Source: CAD feature listing. Evaluate the final solid. Frame: model axes, mm. A direction names the side the tool comes from. Give positions to 0.01 mm unless a question says otherwise; leave off trailing zeros. Write each loop counter-clockwise with the first axis right and the second up, starting at its lowest first coordinate (ties: lowest second). Pieces come first, ordered by that corner, then holes. Notation, with made-up numbers: (-23, -11) - (-11, -11) arc R9 ccw to (-11, -7) - close; hole circle Ø2 at (64, -3.75). An arc over 180 degrees is marked (long way). One line per question, with ' | ' between items. Start each with the question number.
(1) Ray query, line 1 (Y direction, x = 15, z = 4); line 2 (X direction, y = 5, z = 6.25); line 3 (X direction, y = 12, z = 4). Return the intervals inside material, ascending. Write a range as [from, to].
(2) Section B-B, the plane x = 55. Return loops of the section in (y, z), plus the area to 3 significant figures.
(3) Section D-D, the plane y = 12.5. Return loops of the section in (x, z), plus the area to 3 significant figures.
(4) Section C-C, the plane y = 49. Return loops of the section in (x, z).
(5) Pin query (flat end, axial travel): pin 1 (19 mm diameter, centred on x = 33.93, y = 49, fed in from -Z); pin 2 (16 mm diameter, centred on x = 55, y = 15, fed in from -Z). Return the tip coordinate at first contact, or that it passes through.
(6) Access query for faces 4 (the flat face through (31, 8, 2)), 5 (the flat face through (17, 10, 8)), 6 (the cylindrical face through (55, 31, 2)). Directions: +Z, -Z, +X, -X, +Y, -Y. A direction counts if a zero-diameter tool reaches every point of the face in a straight line with its end or side. Return the directions, or none.
(7) Section A-A, the plane z = 1.5. Return loops of the section in (x, y).
(8) Draft query along X for faces 1 (the flat face through (-1, 27, 7)), 2 (the flat face through (34, 70, 8)), 3 (the flat face through (39, 7, 2)). Return one class per face: +X half, -X half, draft (parallel to the pull), parting line (faces both ways), or undercut.
```python
from build123d import *

# Parameters (mm, degrees)
SKETCH1_W               = 70
SKETCH1_H               = 70
BOSS_EXTRUDE1_DEPTH     = 10
SKETCH2_R               = 12
SKETCH2_R_2             = 2
SKETCH2_R_3             = 11.5
CUT_EXTRUDE1_DEPTH      = 10
SKETCH3_W               = 10
SKETCH3_H               = 70
BOSS_EXTRUDE2_DEPTH     = 15
SKETCH4_W               = 10
SKETCH4_H               = 70
BOSS_EXTRUDE3_DEPTH     = 15
SKETCH5_R               = 11.5
SKETCH5_R_2             = 4
BOSS_EXTRUDE4_DEPTH     = 2
SKETCH6_R               = 1.5
SKETCH6_R_2             = 1.648708122
CUT_EXTRUDE3_DEPTH      = 10
BOSS_EXTRUDE5_START     = -10
SKETCH7_R               = 11.986708095
SKETCH7_R_2             = 2
BOSS_EXTRUDE5_DEPTH     = 10
SKETCH8_R               = 12
CUT_EXTRUDE4_DEPTH      = 10
SKETCH9_R               = 2
CUT_EXTRUDE5_DEPTH      = 10
CUT_EXTRUDE7_DEPTH      = 5
SKETCH15_W              = 14
SKETCH15_H              = 70
CUT_EXTRUDE8_DEPTH      = 5
CUT_EXTRUDE9_DEPTH      = 19
CUT_EXTRUDE9_DEPTH_BACK = 48
SKETCH16_R              = 1.5
SKETCH17_R              = 5
CUT_EXTRUDE10_DEPTH     = 19
SKETCH18_R              = 16.289174866
SKETCH18_R_2            = 12
BOSS_EXTRUDE6_DEPTH     = 5


with BuildPart() as part:
    # Sketch1 → Boss-Extrude1 (new body)
    with BuildSketch(Plane.XY):
        with Locations((35, 35)):
            Rectangle(SKETCH1_W, SKETCH1_H)
    extrude(amount=BOSS_EXTRUDE1_DEPTH)

    # Sketch2 → Cut-Extrude1 (cut)
    with BuildSketch(Plane.XY.offset(10)):
        with Locations((35, 49)):
            Circle(SKETCH2_R)
        with Locations((19.5, 65)):
            Circle(SKETCH2_R_2)
        with Locations((50.5, 65)):
            Circle(SKETCH2_R_2)
        with Locations((19.5, 34)):
            Circle(SKETCH2_R_2)
        with Locations((50.5, 34)):
            Circle(SKETCH2_R_2)
        with Locations((15, 15)):
            Circle(SKETCH2_R_3)
        with Locations((55, 15)):
            Circle(SKETCH2_R_3)
    extrude(amount=-CUT_EXTRUDE1_DEPTH, mode=Mode.SUBTRACT)

    # Sketch3 → Boss-Extrude2 (add)
    with BuildSketch(Plane.ZY):
        with Locations((5, 35)):
            Rectangle(SKETCH3_W, SKETCH3_H)
    extrude(amount=BOSS_EXTRUDE2_DEPTH)

    # Sketch4 → Boss-Extrude3 (add)
    with BuildSketch(Plane(origin=(70, 0, 0), x_dir=(0, 0, -1), z_dir=(1, 0, 0))):
        with Locations((-5, 35)):
            Rectangle(SKETCH4_W, SKETCH4_H)
    extrude(amount=BOSS_EXTRUDE3_DEPTH)

    # Sketch5 → Boss-Extrude4 (add)
    # profile 1 of 2: a face of its own
    with BuildSketch(Plane.XY.offset(10)):
        with Locations((15, 15)):
            Circle(SKETCH5_R)
        with Locations((15, 15)):
            Circle(SKETCH5_R_2, mode=Mode.SUBTRACT)
    # profile 2 of 2: a face of its own
    with BuildSketch(Plane.XY.offset(10)):
        with Locations((55, 15)):
            Circle(SKETCH5_R)
        with Locations((55, 15)):
            Circle(SKETCH5_R_2, mode=Mode.SUBTRACT)
    extrude(amount=-BOSS_EXTRUDE4_DEPTH)

    # Sketch6 → Cut-Extrude3 (cut)
    with BuildSketch(Plane(origin=(0, 0, 0), x_dir=(-1, 0, 0), z_dir=(0, 0, -1))):
        with Locations((-80, 65)):
            Circle(SKETCH6_R)
        with Locations((-80, 5)):
            Circle(SKETCH6_R)
        with Locations((10, 65)):
            Circle(SKETCH6_R_2)
        with Locations((10, 5)):
            Circle(SKETCH6_R)
    extrude(amount=-CUT_EXTRUDE3_DEPTH, mode=Mode.SUBTRACT)

    # Sketch7 → Boss-Extrude5 (add)
    with BuildSketch(Plane(origin=(0, 0, 0), x_dir=(-1, 0, 0), z_dir=(0, 0, -1)).offset(BOSS_EXTRUDE5_START)):
        with Locations((-35, 49)):
            Circle(SKETCH7_R)
        with Locations((-50.5, 65)):
            Circle(SKETCH7_R_2)
        with Locations((-19.5, 65)):
            Circle(SKETCH7_R_2)
        with Locations((-19.5, 34)):
            Circle(SKETCH7_R_2)
        with Locations((-50.5, 34)):
            Circle(SKETCH7_R_2)
    extrude(amount=BOSS_EXTRUDE5_DEPTH)


with BuildPart() as boss_extrude5_piece_1:
    # of the separate pieces the step leaves, piece 1, a body of its own (boss_extrude5_pieces)
    add(part.part.solids().sort_by_distance((-15, 0, 0))[0])


with BuildPart() as boss_extrude5_piece_2:
    # of the separate pieces the step leaves, piece 2, a body of its own (boss_extrude5_pieces)
    add(part.part.solids().sort_by_distance((23.013291905, 49, 10))[0])


with BuildPart() as cut_extrude4_tool:
    # Sketch8 → Cut-Extrude4 (new body)
    with BuildSketch(Plane(origin=(0, 0, 0), x_dir=(-1, 0, 0), z_dir=(0, 0, -1))):
        with Locations((-33.928692494, 49)):
            Circle(SKETCH8_R)
    extrude(amount=-CUT_EXTRUDE4_DEPTH)


with BuildPart() as boss_extrude5_piece_1_1:
    add(boss_extrude5_piece_1.part)

    # Cut-Extrude4: cut by cut_extrude4_tool
    add(cut_extrude4_tool.part, mode=Mode.SUBTRACT)

    # Sketch9 → Cut-Extrude5 (cut)
    with BuildSketch(Plane(origin=(0, 0, 0), x_dir=(-1, 0, 0), z_dir=(0, 0, -1))):
        with Locations((-49.428692494, 64.5)):
            Circle(SKETCH9_R)
        with Locations((-49.428692494, 33.5)):
            Circle(SKETCH9_R)
        with Locations((-18.428692494, 33.5)):
            Circle(SKETCH9_R)
        with Locations((-18.428692494, 64.5)):
            Circle(SKETCH9_R)
    extrude(amount=-CUT_EXTRUDE5_DEPTH, mode=Mode.SUBTRACT)


with BuildPart() as boss_extrude5_piece_2_1:
    add(boss_extrude5_piece_2.part)

    # Cut-Extrude4: cut by cut_extrude4_tool
    add(cut_extrude4_tool.part, mode=Mode.SUBTRACT)


with BuildPart() as cut_extrude7_tool:
    # Sketch14 → Cut-Extrude7 (new body)
    with BuildSketch(Plane(origin=(0, 0, 0), x_dir=(-1, 0, 0), z_dir=(0, 0, -1))):
        with BuildLine():
            Line((-85, 0), (-85, 70))
            Line((-85, 70), (15, 70))
            Line((15, 70), (15, 0))
            Line((15, 0), (1, 0))
            Line((1, 0), (1, 15))
            ThreePointArc((1, 15), (-15, 31), (-31, 15))
            Line((-31, 15), (-31, 0))
            Line((-31, 0), (-39, 0))
            Line((-39, 0), (-39, 15))
            ThreePointArc((-39, 15), (-55, 31), (-71, 15))
            Line((-71, 15), (-71, 0))
            Line((-71, 0), (-85, 0))
        make_face()
    extrude(amount=-CUT_EXTRUDE7_DEPTH)


with BuildPart() as boss_extrude5_piece_1_2:
    add(boss_extrude5_piece_1_1.part)

    # Cut-Extrude7: cut by cut_extrude7_tool
    add(cut_extrude7_tool.part, mode=Mode.SUBTRACT)

    # Sketch15 → Cut-Extrude8 (cut)
    with BuildSketch(Plane(origin=(0, 0, 5), x_dir=(-1, 0, 0), z_dir=(0, 0, -1))):
        with Locations((-78, 35)):
            Rectangle(SKETCH15_W, SKETCH15_H)
        with Locations((8, 35)):
            Rectangle(SKETCH15_W, SKETCH15_H)
    extrude(amount=-CUT_EXTRUDE8_DEPTH, mode=Mode.SUBTRACT)

    # Sketch16 → Cut-Extrude9 (cut, two sides: drawn at the far end of the back side and taken through both)
    with BuildSketch(Plane(origin=(0, 0, 5), x_dir=(-1, 0, 0), z_dir=(0, 0, -1)).offset(-CUT_EXTRUDE9_DEPTH_BACK)):
        with Locations((-66, 65)):
            Circle(SKETCH16_R)
        with Locations((-66, 5)):
            Circle(SKETCH16_R)
        with Locations((-4, 5)):
            Circle(SKETCH16_R)
        with Locations((-4, 65)):
            Circle(SKETCH16_R)
    extrude(amount=CUT_EXTRUDE9_DEPTH + CUT_EXTRUDE9_DEPTH_BACK, mode=Mode.SUBTRACT)

    # Sketch17 → Cut-Extrude10 (cut)
    with BuildSketch(Plane(origin=(0, 0, 8), x_dir=(-1, 0, 0), z_dir=(0, 0, -1))):
        with Locations((-15, 15)):
            Circle(SKETCH17_R)
        with Locations((-55, 15)):
            Circle(SKETCH17_R)
    extrude(amount=-CUT_EXTRUDE10_DEPTH, mode=Mode.SUBTRACT)



with BuildPart() as boss_extrude5_piece_2_2:
    add(boss_extrude5_piece_2_1.part)

    # Cut-Extrude7: cut by cut_extrude7_tool
    add(cut_extrude7_tool.part, mode=Mode.SUBTRACT)


with BuildPart() as boss_extrude5_piece_1_3:
    add(boss_extrude5_piece_1_2.part)

    add(boss_extrude5_piece_2_2.part)  # Boss-Extrude6 merges Boss-Extrude5 piece 2
    # Sketch18 → Boss-Extrude6 (add)
    with BuildSketch(Plane(origin=(0, 0, 5), x_dir=(-1, 0, 0), z_dir=(0, 0, -1))):
        with Locations((-33.928692494, 49)):
            Circle(SKETCH18_R)
        with Locations((-33.928692494, 49)):
            Circle(SKETCH18_R_2, mode=Mode.SUBTRACT)
    extrude(amount=-BOSS_EXTRUDE6_DEPTH)


solid = boss_extrude5_piece_1_3.part
```
Check sheet entries:
1) line 1: [0, 3.5], [26.5, 31] | line 2: [-1, 2.5], [5.5, 9.32], [20.68, 49.32], [60.68, 64.5], [67.5, 71] | line 3: [-1, 3.9], [26.1, 31], [39, 43.9], [66.1, 71]
2) outline: (0, 0) - (3.5, 0) - (3.5, 8) - (10, 8) - (10, 10) - (0, 10) - close; (20, 8) - (26.5, 8) - (26.5, 0) - (31, 0) - (31, 5) - (70, 5) - (70, 10) - (20, 10) - close | area: 301 mm²
3) outline: (-1, 0) - (3.78, 0) - (3.78, 8) - (10.67, 8) - (10.67, 10) - (-1, 10) - close; (19.33, 8) - (26.22, 8) - (26.22, 0) - (31, 0) - (31, 5) - (39, 5) - (39, 0) - (43.78, 0) - (43.78, 8) - (50.67, 8) - (50.67, 10) - (19.33, 10) - close; (59.33, 8) - (66.22, 8) - (66.22, 0) - (71, 0) - (71, 10) - (59.33, 10) - close | area: 286 mm²
4) outline: (-1, 5) - (21.93, 5) - (21.93, 10) - (-1, 10) - close; (45.93, 5) - (71, 5) - (71, 10) - (45.93, 10) - close
5) pin 1: through | pin 2: z = 8
6) face 4: -Z, +Y, -Y | face 5: -Z | face 6: -Z, +Y
7) outline: (-1, 0) - (31, 0) - (31, 15) arc R16 ccw to (-1, 15) - close; (39, 0) - (71, 0) - (71, 15) arc R16 ccw to (39, 15) - close; hole circle Ø3 at (4, 5); hole circle Ø23 at (15, 15); hole circle Ø23 at (55, 15); hole circle Ø3 at (66, 5)
8) face 1: -X half | face 2: draft | face 3: undercut
